from build123d import *

# Parameters (mm, degrees)
SKETCH1_W                  = 80.3
SKETCH1_H                  = 66
BOSS_EXTRUDE1_DEPTH        = 3
FILLET1_R                  = 3.5
SKETCH2_W                  = 72.4
SKETCH2_H                  = 45
CUT_EXTRUDE1_DEPTH         = 4
SKETCH3_W                  = 15
SKETCH3_H                  = 30
SKETCH3_W_2                = 33
SKETCH3_H_2                = 18
SKETCH3_W_3                = 39
SKETCH3_H_3                = 18.5
CUT_EXTRUDE2_DEPTH         = 4
F_3_2_3_2_DIAMETER_HOLE1_D = 3.2
SKETCH9_W                  = 72.9
SKETCH9_H                  = 45.5
SKETCH9_W_2                = 33.5
SKETCH9_H_2                = 18.5
SKETCH9_W_3                = 39.5
SKETCH9_H_3                = 19
SKETCH9_W_4                = 15.5
SKETCH9_H_4                = 30.5
CUT_EXTRUDE3_DEPTH         = 4


with BuildPart() as part:
    # Sketch1 → Boss-Extrude1 (new body)
    with BuildSketch(Plane.XY):
        Polygon((-18, -20), (60.3, -20), (80.3, 0), (0, 0), (0, 66), (-18, 48), align=None)
        with Locations((40.15, 33)):
            Rectangle(SKETCH1_W, SKETCH1_H)
    extrude(amount=BOSS_EXTRUDE1_DEPTH)

    # Fillet1
    fillet1_edges = [part.edges().sort_by_distance(p)[0] for p in [
        (60.3, -20, 1.5),
        (-18, -20, 1.5),
        (-18, 48, 1.5),
        (0, 66, 1.5),
        (80.3, 66, 1.5),
        (80.3, 0, 1.5),
    ]]
    fillet(fillet1_edges, radius=FILLET1_R)

    # Sketch2 → Cut-Extrude1 (cut, through all)
    with BuildSketch(Plane.XY.offset(3)):
        with Locations((39.2, 33)):
            Rectangle(SKETCH2_W, SKETCH2_H)
    extrude(amount=-CUT_EXTRUDE1_DEPTH, mode=Mode.SUBTRACT)

    # Sketch3 → Cut-Extrude2 (cut, through all)
    with BuildSketch(Plane.XY.offset(3)):
        with BuildLine():
            Line((-3, 47.3), (-17.918753974, 47.3))
            ThreePointArc((-17.918753974, 47.3), (-17.979629212, 46.927320889), (-18, 46.550252532))
            Line((-18, 46.550252532), (-18, 36.5))
            Line((-18, 36.5), (-3, 36.5))
            Line((-3, 36.5), (-3, 47.3))
        make_face()
        with Locations((-7.5, 19.5)):
            Rectangle(SKETCH3_W, SKETCH3_H)
        with Locations((43.5, -8)):
            Rectangle(SKETCH3_W_2, SKETCH3_H_2)
        with Locations((4.5, -7.75)):
            Rectangle(SKETCH3_W_3, SKETCH3_H_3)
        Polygon((67.242640687, -0.329437252), (63, -4.572077939), (67.242640687, -8.814718626), (71.485281374, -4.572077939), align=None)
    extrude(amount=-CUT_EXTRUDE2_DEPTH, mode=Mode.SUBTRACT)

    # 3.2 _3.2_ Diameter Hole1 (through all)
    with Locations(Plane.XY.offset(3)):
        with Locations((7, 59), (73.3, 59), (73.3, 7), (7, 7)):
            Hole(F_3_2_3_2_DIAMETER_HOLE1_D / 2)

    # Sketch9 → Cut-Extrude3 (cut, through all)
    with BuildSketch(Plane.XY.offset(3)):
        with Locations((39.2, 33)):
            Rectangle(SKETCH9_W, SKETCH9_H)
        with Locations((43.5, -8)):
            Rectangle(SKETCH9_W_2, SKETCH9_H_2)
        Polygon((67.242640687, -9.168272016), (71.838834765, -4.572077939), (67.242640687, 0.024116139), (62.646446609, -4.572077939), align=None)
        with Locations((4.5, -7.75)):
            Rectangle(SKETCH9_W_3, SKETCH9_H_3)
        with Locations((-7.5, 19.5)):
            Rectangle(SKETCH9_W_4, SKETCH9_H_4)
    extrude(amount=-CUT_EXTRUDE3_DEPTH, mode=Mode.SUBTRACT)


solid = part.part
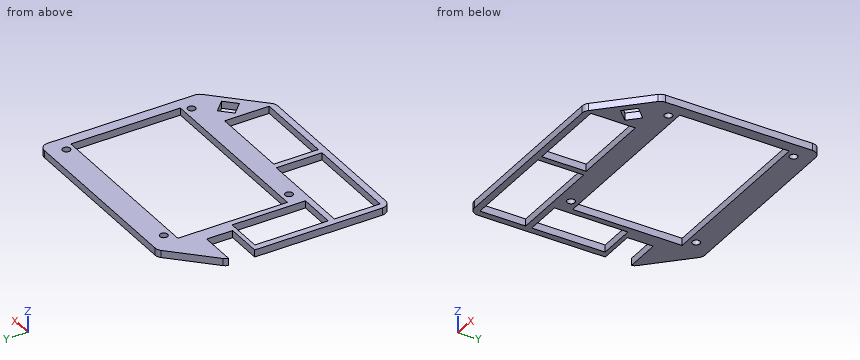
For this review, take the finished solid that the model builds, in its own axes (mm). Round coordinates to 2 decimals unless told otherwise and drop trailing zeros. Loops run counter-clockwise (first coordinate to the right, second up) from the corner with the lowest first, then second, coordinate; pieces in that order, holes last. Notation, with made-up numbers: (-4.75, 53) - (9.25, 53) arc R19 cw to (9.25, 83) - close; hole circle Ø9 at (17, 13.5). An arc over 180 degrees is marked (long way). One line per question, with ' | ' between items.
Q1. Take a section at B-B (y = 7). Give the boundary of the cut face in (x, z).
Taken from the geometry:
outline: (-18, 0) - (-15.25, 0) - (-15.25, 3) - (-18, 3) - close; (0.25, 0) - (5.4, 0) - (5.4, 3) - (0.25, 3) - close; (8.6, 0) - (71.7, 0) - (71.7, 3) - (8.6, 3) - close; (74.9, 0) - (80.3, 0) - (80.3, 3) - (74.9, 3) - close
Q2. For line 1 along Y through (x, z) = (38.5, 1); line 2 along X through (y, z) = (30.5, 1); line 3 along Y through (x, z) = (17, 2.95), list the stretches that pass through material, from the lowest coordinate up. Write a range as [from, to].
Taken from the geometry:
line 1: y = [-20, -17.25], [1.25, 10.25], [55.75, 66] | line 2: x = [-18, -15.25], [0.25, 2.75], [75.65, 80.3] | line 3: y = [-20, -17.25], [1.75, 10.25], [55.75, 66]
Q3. Take a section at C-C (x = 73.3). Give the boundary of the cut face in (y, z), and give its area (3 significant figures).
Taken from the geometry:
outline: (-7, 0) - (5.4, 0) - (5.4, 3) - (-7, 3) - close; (8.6, 0) - (10.25, 0) - (10.25, 3) - (8.6, 3) - close; (55.75, 0) - (57.4, 0) - (57.4, 3) - (55.75, 3) - close; (60.6, 0) - (66, 0) - (66, 3) - (60.6, 3) - close | area: 63.3 mm²
Q4. Take a section at A-A (x = 7). Give the boundary of the cut face in (y, z).
Taken from the geometry:
outline: (-20, 0) - (-17.25, 0) - (-17.25, 3) - (-20, 3) - close; (1.75, 0) - (5.4, 0) - (5.4, 3) - (1.75, 3) - close; (8.6, 0) - (10.25, 0) - (10.25, 3) - (8.6, 3) - close; (55.75, 0) - (57.4, 0) - (57.4, 3) - (55.75, 3) - close; (60.6, 0) - (66, 0) - (66, 3) - (60.6, 3) - close
Q5. For pin 1 (3 mm diameter, centred on x = 73.3, y = 7, fed in from +Z); pin 2 (1.5 mm diameter, centred on x = -1.5, z = 1.5, fed in from +Y); pin 3 (1.5 mm diameter, centred on y = -4, z = 2, fed in from +X), all flat-tipped, find the tip position at first contact; note any pin that passes through.
Taken from the geometry:
pin 1: passes through | pin 2: stops at y = 65.22 | pin 3: stops at x = 77.05
Q6. Take a section at D-D (y = 59). Give the boundary of the cut face in (x, z), and give its area (3 significant figures).
Taken from the geometry:
outline: (-7, 0) - (5.4, 0) - (5.4, 3) - (-7, 3) - close; (8.6, 0) - (71.7, 0) - (71.7, 3) - (8.6, 3) - close; (74.9, 0) - (80.3, 0) - (80.3, 3) - (74.9, 3) - close | area: 243 mm²
